Part model, mm, in its own coordinate system. Face numbers are marked on the shaded views. A direction names the side the tool comes from. Round coordinates to 2 decimals unless told otherwise and drop trailing zeros. Order: outer loops, then holes, each group sorted by start corner. A loop starts at its lowest first (then second) coordinate and runs counter-clockwise, first axis right, second up. Notation, with made-up numbers: (-14, 43) -> (17, 43) arc R17 cw to (17, 47) -> close; hole circle Ø2 at (-33, 83.5). An arc over 180 degrees is marked (long way). Use CSV: the item, a comma, the result in double quotes.
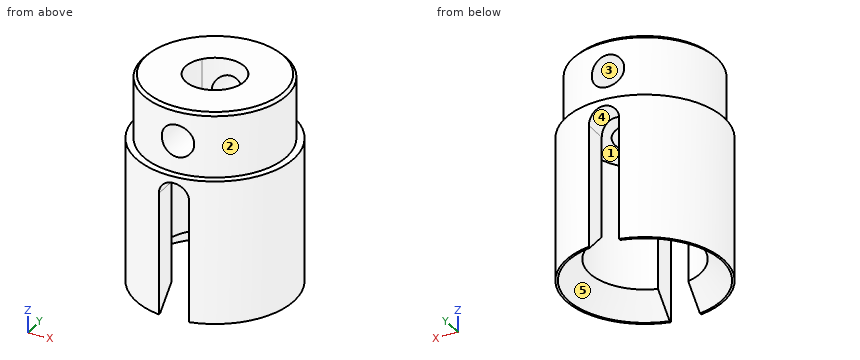
```python
from build123d import *

# Parameters (mm, degrees)
SKETCH_1_R           = 11
EXTRUDE_1_DEPTH      = 29
SKETCH_2_OUTSIDE_W   = 32.506
SKETCH_2_OUTSIDE_H   = 32.506
SKETCH_2_OUTSIDE_R   = 10
CUT_EXTRUDE_1_DEPTH  = 9
SKETCH_3_R           = 7.7
CUT_EXTRUDE_2_DEPTH  = 20
SKETCH_4_R           = 2.1
CUT_EXTRUDE_3_DEPTH  = 25
CHAMFER_1_SIZE       = 3
EXTRUDE_START        = 10
SKETCH_5_R           = 10
EXTRUDE_2_DEPTH      = 10
CUT_EXTRUDE_5_DEPTH  = 19
CUT_EXTRUDE_6_DEPTH  = 19
CHAMFER_2_SIZE       = 0.4
SKETCH_12_R          = 10
CUT_EXTRUDE_9_DEPTH  = 10
SKETCH_13_R          = 4.1
CUT_EXTRUDE_10_DEPTH = 9
SKETCH_14_R          = 2.25
CUT_EXTRUDE_11_DEPTH = 25
CHAMFER_3_SIZE       = 0.4


with BuildPart() as part:
    # 草图1 → 凸台-拉伸1 (new body)
    with BuildSketch(Plane.XY):
        with Locations(Location((0, 0, 0), (0, 0, 180))):
            Circle(SKETCH_1_R)
    extrude(amount=EXTRUDE_1_DEPTH)

    # 草图2 outside → 切除-拉伸1 (cut)
    with BuildSketch(Plane.XY.offset(29)):
        Rectangle(SKETCH_2_OUTSIDE_W, SKETCH_2_OUTSIDE_H)
        Circle(SKETCH_2_OUTSIDE_R, mode=Mode.SUBTRACT)
    extrude(amount=-CUT_EXTRUDE_1_DEPTH, mode=Mode.SUBTRACT)

    # 草图3 → 切除-拉伸2 (cut)
    with BuildSketch(Plane(origin=(0, 0, 0), x_dir=(-1, 0, 0), z_dir=(0, 0, -1))):
        Circle(SKETCH_3_R)
    extrude(amount=-CUT_EXTRUDE_2_DEPTH, mode=Mode.SUBTRACT)

    # 草图4 → 切除-拉伸3 (cut, symmetric)
    with BuildSketch(Plane(origin=(0, 0, 0), x_dir=(1, 0, 0), z_dir=(0, 1, 0))):
        with BuildLine():
            Line((-2.1, 0), (-2.1, -17))
            ThreePointArc((-2.1, -17), (0, -14.9), (2.1, -17))
            Line((2.1, -17), (2.1, 0))
            Line((2.1, 0), (-2.1, 0))
        make_face()
        with Locations((0, -17)):
            Circle(SKETCH_4_R)
    extrude(amount=CUT_EXTRUDE_3_DEPTH, both=True, mode=Mode.SUBTRACT)

    # 倒角1
    chamfer_1_edges = [part.edges().sort_by_distance(p)[0] for p in [
        (7.7, 0, 0),
        (-6.142475071, -4.643274706, 0),
    ]]
    chamfer(chamfer_1_edges, length=CHAMFER_1_SIZE)

    # 草图5 → 凸台-拉伸2 (add)
    with BuildSketch(Plane.XY.offset(29).offset(EXTRUDE_START)):
        Circle(SKETCH_5_R)
    extrude(amount=-EXTRUDE_2_DEPTH)

    # 草图6 → 切除-拉伸5 (cut)
    with BuildSketch(Plane.XY.offset(39)):
        with BuildLine():
            Line((3.122498999, 2.5), (-3.122498999, 2.5))
            ThreePointArc((-3.122498999, 2.5), (-1.324764885, -3.774254628), (4, 0))
            ThreePointArc((4, 0), (3.774254628, 1.324764885), (3.122498999, 2.5))
        make_face()
    extrude(amount=-CUT_EXTRUDE_5_DEPTH, mode=Mode.SUBTRACT)

    # 草图7 → 切除-拉伸6 (cut)
    with BuildSketch(Plane.XY.offset(39)):
        with BuildLine():
            Line((3.170173497, 2.6), (-3.170173497, 2.6))
            ThreePointArc((-3.170173497, 2.6), (0, -4.1), (3.170173497, 2.6))
        make_face()
    extrude(amount=-CUT_EXTRUDE_6_DEPTH, mode=Mode.SUBTRACT)

    # 倒角2
    chamfer_2_edges = [part.edges().sort_by_distance(p)[0] for p in [
        (0, -4.1, 39),
        (0, 2.6, 39),
    ]]
    chamfer(chamfer_2_edges, length=CHAMFER_2_SIZE)

    # 草图12 → 切除-拉伸9 (cut)
    with BuildSketch(Plane.XY.offset(39)):
        Circle(SKETCH_12_R)
    extrude(amount=-CUT_EXTRUDE_9_DEPTH, mode=Mode.SUBTRACT)

    # 草图13 → 切除-拉伸10 (cut)
    with BuildSketch(Plane.XY.offset(29)):
        Circle(SKETCH_13_R)
    extrude(amount=-CUT_EXTRUDE_10_DEPTH, mode=Mode.SUBTRACT)

    # 草图14 → 切除-拉伸11 (cut, symmetric)
    with BuildSketch(Plane(origin=(0, 0, 0), x_dir=(1, 0, 0), z_dir=(0, 1, 0))):
        with Locations(Location((0, -24.5, 0), (0, 0, 270))):
            Circle(SKETCH_14_R)
    extrude(amount=CUT_EXTRUDE_11_DEPTH, both=True, mode=Mode.SUBTRACT)

    # 倒角3
    chamfer_3_edges = [part.edges().sort_by_distance(p)[0] for p in [
        (-10, 0, 29),
    ]]
    chamfer(chamfer_3_edges, length=CHAMFER_3_SIZE)


solid = part.part
```
(1) Drop flat-ended pins along their axis: P1, Ø1, axis at y = -9.5, z = 6.5, coming from the +X side; P2, Ø3.5, axis at x = 0, z = 24.5, coming from the -Y side; P3, Ø3.5, axis at y = 8.5, z = 7, coming from the -X side; P4, Ø10, axis at y = 7.5, z = 3.5, coming from the -X side. Give the stop position or say it passes through.
Reply:
P1,"x = 6.32"
P2,"through"
P3,"x = -8.69"
P4,"x = -10.71"
(2) Cut at B-B, the plane x = 0. Give the cut face in (y, z), then the cut area to 3 significant figures.
Reply:
outline,"(-11, 19.1) -> (-7.7, 19.1) -> (-7.7, 20) -> (-4.1, 20) -> (-4.1, 22.25) -> (-10, 22.25) -> (-10, 20) -> (-11, 20) -> close; (-10, 26.75) -> (-4.1, 26.75) -> (-4.1, 29) -> (-9.6, 29) -> (-10, 28.6) -> close; (4.1, 20) -> (7.7, 20) -> (7.7, 19.1) -> (11, 19.1) -> (11, 20) -> (10, 20) -> (10, 22.25) -> (4.1, 22.25) -> close; (4.1, 26.75) -> (10, 26.75) -> (10, 28.6) -> (9.6, 29) -> (4.1, 29) -> close"
area,"58.9 mm2"
(3) Cut at A-A, the plane z = 8.75. Give the cut face in (x, y), then the cut area to 3 significant figures.
Reply:
outline,"(-2.1, -10.8) -> (-2.1, -7.41) arc R7.7 cw to (-2.1, 7.41) -> (-2.1, 10.8) arc R11 ccw to start; (2.1, -10.8) arc R11 ccw to (2.1, 10.8) -> (2.1, 7.41) arc R7.7 cw to (2.1, -7.41) -> close"
area,"166 mm2"
(4) Cut at D-D, the plane z = 21. Give the cut face in (x, y).
Reply:
outline,"circle Ø20 at (0, 0); hole circle Ø8.2 at (0, 0)"
(5) Probe probe 1 along Z at (x, y) = (0, 6); probe 2 along Y at (x, z) = (1.75, 27); probe 3 along X at (y, z) = (3.25, 5.5). List the from-to ranges inside material, lowest first. Write a range as [from, to].
Reply:
probe 1,"[20, 22.25], [26.75, 29]"
probe 2,"[-9.85, -3.71], [3.71, 9.85]"
probe 3,"[-10.51, -6.98], [6.98, 10.51]"
(6) Cut at C-C, the plane y = 0. Give the cut face in (x, z).
Reply:
outline,"(-11, 0) -> (-10.7, 0) -> (-7.7, 3) -> (-7.7, 20) -> (-4.1, 20) -> (-4.1, 29) -> (-9.6, 29) -> (-10, 28.6) -> (-10, 20) -> (-11, 20) -> close; (4.1, 20) -> (7.7, 20) -> (7.7, 3) -> (10.7, 0) -> (11, 0) -> (11, 20) -> (10, 20) -> (10, 28.6) -> (9.6, 29) -> (4.1, 29) -> close"
(7) Pull direction Y, two halves, no side cores. Call the marked faces 1, 2 and 3: released by +Y, released by -Y, zero draft, split by the parting line, or undercut.
Reply:
face 1,"undercut"
face 2,"split by the parting line"
face 3,"zero draft"
(8) Which spindle directions (+Z, -Z, +X, -X, +Y, -Y) get a long thin tool onto all of the face, cutting with end or side? Do the marked faces 4 and 5. Say none if no direction does.
Reply:
face 4,"-Z, +Y, -Y"
face 5,"-Z"
